```python
from build123d import *

# Parameters (mm, degrees)
CUT_EXTRUDE_START        = 7
SKETCH_9_R               = 3
SKETCH_9_R_2             = 1.5
CUT_EXTRUDE_1_DEPTH      = 5
CUT_EXTRUDE_START_2      = 55
CUT_EXTRUDE_9_DEPTH      = 43
CUT_EXTRUDE_11_DEPTH     = 74.972968036
EXTRUDE_START            = -8
EXTRUDE_17_DEPTH         = 8
SKETCH_26_R              = 2
CUT_EXTRUDE_12_DEPTH     = 5
PATTERN_CIRCULAR_3_COUNT = 4
PATTERN_CIRCULAR_3_ANGLE = 180
SKETCH_22_R              = 2.5
EXTRUDE_19_DEPTH         = 7
SKETCH_28_R              = 1.25
CUT_EXTRUDE_13_DEPTH     = 5


with BuildPart() as part:
    # Эскиз6 → Повернуть1 (revolve)
    with BuildSketch(Plane(origin=(0, 0, 0), x_dir=(0, 0, -1), z_dir=(1, 0, 0))):
        Polygon((26, 0), (44, 0), (44, 52), (39, 52), (39, 12), (0, 12), (0, 7), (26, 7), align=None)
    revolve(axis=Axis((0, 0, 0), (0, 1, 0)))

    # Эскиз9 → Вырез-Вытянуть1 (cut)
    with BuildSketch(Plane(origin=(0, 0, 0), x_dir=(1, 0, 0), z_dir=(0, 1, 0)).offset(CUT_EXTRUDE_START)):
        with Locations(Location((0, 0, 0), (0, 0, 270))):
            Circle(SKETCH_9_R)
        with Locations(Location((0, 7, 0), (0, 0, 270))):
            Circle(SKETCH_9_R_2)
        with Locations(Location((7, 0, 0), (0, 0, 270))):
            Circle(SKETCH_9_R_2)
        with Locations(Location((0, -7, 0), (0, 0, 270))):
            Circle(SKETCH_9_R_2)
        with Locations(Location((-7, 0, 0), (0, 0, 270))):
            Circle(SKETCH_9_R_2)
    extrude(amount=CUT_EXTRUDE_1_DEPTH, mode=Mode.SUBTRACT)

    # Эскиз21 → Вырез-Вытянуть9 (cut)
    with BuildSketch(Plane(origin=(0, 0, 0), x_dir=(1, 0, 0), z_dir=(0, 1, 0)).offset(CUT_EXTRUDE_START_2)):
        with BuildLine():
            Line((41.269210876, -15.259496508), (-41.269210876, -15.259496508))
            ThreePointArc((-41.269210876, -15.259496508), (0, -44), (41.269210876, -15.259496508))
        make_face()
    extrude(amount=-CUT_EXTRUDE_9_DEPTH, mode=Mode.SUBTRACT)

    # Эскиз23 → Вырез-Вытянуть11 (cut, through all)
    with BuildSketch(Plane(origin=(0, 12, 0), x_dir=(1, 0, 0), z_dir=(0, 1, 0))):
        with BuildLine():
            Line((-29.373719352, -32.759496508), (29.373719352, -32.759496508))
            ThreePointArc((29.373719352, -32.759496508), (0, -44), (-29.373719352, -32.759496508))
        make_face()
    extrude(amount=-CUT_EXTRUDE_11_DEPTH, mode=Mode.SUBTRACT)

    # Эскиз25 → Бобышка-Вытянуть17 (add)
    with BuildSketch(Plane(origin=(0, 52, 0), x_dir=(1, 0, 0), z_dir=(0, 1, 0)).offset(EXTRUDE_START)):
        with BuildLine():
            ThreePointArc((-38.679487179, -4.989716578), (-34, 0), (-38.679487179, 4.989716578))
            ThreePointArc((-38.679487179, 4.989716578), (-39, 0), (-38.679487179, -4.989716578))
        make_face()
    extrude_17 = extrude(amount=EXTRUDE_17_DEPTH)

    # Эскиз26 → Вырез-Вытянуть12 (cut)
    with BuildSketch(Plane(origin=(0, 52, 0), x_dir=(1, 0, 0), z_dir=(0, 1, 0))):
        with Locations(Location((-39, 0, 0), (0, 0, 270))):
            Circle(SKETCH_26_R)
    cut_extrude_12 = extrude(amount=-CUT_EXTRUDE_12_DEPTH, mode=Mode.SUBTRACT)

    # Круговой массив3: Бобышка-Вытянуть17, Вырез-Вытянуть12 ×4 about axis
    pattern_circular_3_axis = Axis((0, 0, 0), (0, -1, 0))
    add([extrude_17.rotate(pattern_circular_3_axis, i * PATTERN_CIRCULAR_3_ANGLE / (PATTERN_CIRCULAR_3_COUNT - 1)) for i in range(1, PATTERN_CIRCULAR_3_COUNT)])
    add([cut_extrude_12.rotate(pattern_circular_3_axis, i * PATTERN_CIRCULAR_3_ANGLE / (PATTERN_CIRCULAR_3_COUNT - 1)) for i in range(1, PATTERN_CIRCULAR_3_COUNT)], mode=Mode.SUBTRACT)

    # Эскиз22 → Бобышка-Вытянуть19 (add)
    with BuildSketch(Plane.XY.offset(15.259496508)):
        with Locations((-38, 16)):
            Circle(SKETCH_22_R)
        with Locations((-38, 48)):
            Circle(SKETCH_22_R)
        with Locations((38, 48)):
            Circle(SKETCH_22_R)
        with Locations((38, 16)):
            Circle(SKETCH_22_R)
    extrude(amount=-EXTRUDE_19_DEPTH)

    # Эскиз28 → Вырез-Вытянуть13 (cut)
    with BuildSketch(Plane.XY.offset(15.259496508)):
        with Locations((-38, 16)):
            Circle(SKETCH_28_R)
        with Locations((-38, 48)):
            Circle(SKETCH_28_R)
        with Locations((38, 48)):
            Circle(SKETCH_28_R)
        with Locations((38, 16)):
            Circle(SKETCH_28_R)
    extrude(amount=-CUT_EXTRUDE_13_DEPTH, mode=Mode.SUBTRACT)


solid = part.part
```
Here's how the part is built. I have some questions about the finished solid (model axes, mm). A direction names the side the tool comes from. Coordinates: 2 decimals unless noted, no trailing zeros. Loops run counter-clockwise (first coordinate to the right, second up) from the corner with the lowest first, then second, coordinate; pieces in that order, holes last. Notation, with made-up numbers: (-13, 44.25) - (42, 44.25) arc R5 cw to (42, 50.25) - close; hole circle Ø1 at (-34, 42.25). An arc over 180 degrees is marked (long way). Return JSON: item names as keys, results as strings. Group by question number.
Item 1: If we section it at B-B on y = 16: Write out the boundary of the cut face in (x, z).
Item 2: If we section it at A-A on z = -7: Write out the boundary of the cut face in (x, y).
Item 3: If we section it at D-D on x = 19.5: Write out the boundary of the cut face in (y, z) (1 decimal), and give its area (3 significant figures).
Item 4: Will these pins go through, and if not, where does the flat tip stop? P1, Ø2, axis at y = 11.5, z = -23.5, coming from the -X side; P2, Ø8, axis at x = 16, z = -11.5, coming from the -Y side; P3, Ø3, axis at x = -38, y = 48, coming from the +Z side.
Item 5: On a 3-axis mill with a long thin cutter (end or side, diameter ignored), from which of +Z, -Z, +X, -X, +Y, -Y can I reach the whole of each face in a straight line? I mean faces 5 (the face through (15.821, 3.451, 20.633)), 6 (the face through (-35.5, 15.9, 11)), 7 (the face through (39, 32, 15.259)), 8 (the face through (-38.921, 16.845, 12.794)), 9 (the face through (-18.28, 49.54, -32.19)). Say none if no direction works.
Item 6: If we section it at C-C on z = -18.5: Write out the boundary of the cut face in (x, y), and give its area (3 significant figures).
Item 7: I need wall thicknesses on line 1 (Y direction, x = -38, z = 13.05); line 2 (X direction, y = 49.85, z = 0); line 3 (X direction, y = 22.5, z = -1). Which ranges of each line are inside material? Lowest first, please. Write a range as from..to.
Item 8: We'd pull the mould along Z, two halves only. Please class faces 1 (the face through (-35.5, 47.9, 11)), 2 (the face through (-38, 16, 10.259)), 3 (the face through (20, 47, -34)), 4 (the face through (37.84, 49.24, 12.79)): +Z half, -Z half, draft (parallel to the pull), parting line (faces both ways), or undercut.
Calculated:
{
 "1": {"outline": "(-41.27, 15.26) arc R44 ccw (long way) to (41.27, 15.26) - (39.25, 15.26) - (39.25, 10.26) - (36.75, 10.26) - (36.75, 15.26) - (35.5, 15.26) - (35.5, 8.26) - (38.12, 8.26) arc R39 cw (long way) to (-38.12, 8.26) - (-35.5, 8.26) - (-35.5, 15.26) - (-36.75, 15.26) - (-36.75, 10.26) - (-39.25, 10.26) - (-39.25, 15.26) - close"},
 "2": {"outline": "(-43.44, 0) - (-25.04, 0) - (-25.04, 7) - (-1.5, 7) - (-1.5, 12) - (-38.37, 12) - (-38.37, 52) - (-43.44, 52) - close; (1.5, 7) - (25.04, 7) - (25.04, 0) - (43.44, 0) - (43.44, 52) - (38.37, 52) - (38.37, 12) - (1.5, 12) - close"},
 "3": {"outline": "(0, -39.4) - (52, -39.4) - (52, -35.8) - (47, -35.8) - (47, -31.8) - (52, -31.8) - (52, -28.8) - (44, -28.8) - (44, -33.8) - (12, -33.8) - (12, 32.8) - (0, 32.8) - (0, 17.2) - (7, 17.2) - (7, -17.2) - (0, -17.2) - close", "area": "872 mm^2"},
 "4": {"P1": "stops at x = -37.81", "P2": "stops at y = 7", "P3": "stops at z = 15.26"},
 "5": {"face 5": "-Y", "face 6": "none", "face 7": "+Z, +X, -X, +Y", "face 8": "+Z", "face 9": "+Y"},
 "6": {"outline": "(-39.92, 0) - (-18.27, 0) - (-18.27, 7) - (18.27, 7) - (18.27, 0) - (39.92, 0) - (39.92, 52) - (34.33, 52) - (34.33, 12) - (-34.33, 12) - (-34.33, 52) - (-39.92, 52) - close", "area": "1,150 mm^2"},
 "7": {"line 1": "y = 0..14.75, 17.25..46.75, 49.25..52", "line 2": "x = -44..-41, -37..-34, 34..37, 41..44", "line 3": "x = -43.99..-38.99, 38.99..43.99"},
 "8": {"face 1": "undercut", "face 2": "+Z half", "face 3": "undercut", "face 4": "draft"}
}
